Geometry: final body of the model. Coordinates: model frame, mm. Face numbers are marked on the shaded views. A direction names the side the tool comes from. Round coordinates to 2 decimals unless told otherwise and drop trailing zeros. Order: outer loops, then holes, each group sorted by start corner. A loop starts at its lowest first (then second) coordinate and runs counter-clockwise, first axis right, second up. Notation, with made-up numbers: (88, 80) -> (117, 80) arc R8 ccw to (117, 89) -> close; hole circle Ø8 at (41.25, -14.75). An arc over 180 degrees is marked (long way). Put each result on its own line as item: value.
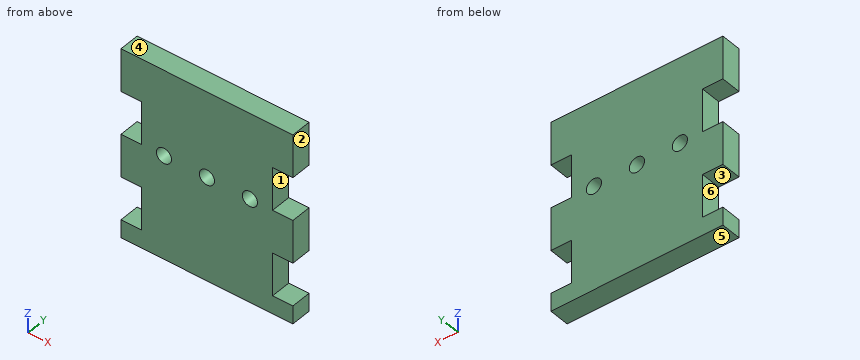
```python
from build123d import *

# Parameters (mm, degrees)
SKETCH1_W            = 50.8
SKETCH1_H            = 56.134
MAIN_DEPTH           = 6
SKETCH2_W            = 6
SKETCH2_H            = 12.7
ACRYLIC_MOUNTS_DEPTH = 39.326446339
SKETCH3_R            = 2.2479
CUT_EXTRUDE1_DEPTH   = 39.326446339


with BuildPart() as part:
    # Sketch1 → Main (new body)
    with BuildSketch(Plane(origin=(0, 0, 0), x_dir=(1, 0, 0), z_dir=(0, 1, 0))):
        Rectangle(SKETCH1_W, SKETCH1_H)
    extrude(amount=MAIN_DEPTH)

    # Sketch2 → Acrylic Mounts (cut, through all)
    with BuildSketch(Plane(origin=(0, 6, 0), x_dir=(1, 0, 0), z_dir=(0, 1, 0))):
        with Locations((-22.4, -9.017)):
            Rectangle(SKETCH2_W, SKETCH2_H)
        with Locations((-22.4, 16.383)):
            Rectangle(SKETCH2_W, SKETCH2_H)
        with Locations((22.4, 16.383)):
            Rectangle(SKETCH2_W, SKETCH2_H)
        with Locations((22.4, -9.017)):
            Rectangle(SKETCH2_W, SKETCH2_H)
    extrude(amount=-ACRYLIC_MOUNTS_DEPTH, mode=Mode.SUBTRACT)

    # Sketch3 → Cut-Extrude1 (cut, through all)
    with BuildSketch(Plane(origin=(0, 0, 0), x_dir=(-1, 0, 0), z_dir=(0, -1, 0))):
        with Locations(Location((12.7, -2.667, 0), (0, 0, 90))):
            Circle(SKETCH3_R)
        with Locations(Location((-12.7, -2.667, 0), (0, 0, 90))):
            Circle(SKETCH3_R)
        with Locations(Location((0, -2.667, 0), (0, 0, 90))):
            Circle(SKETCH3_R)
    extrude(amount=-CUT_EXTRUDE1_DEPTH, mode=Mode.SUBTRACT)


solid = part.part
```
1. Draft query along Z for the marked faces 4, 5 and 6. Return one class per face: +Z half, -Z half, draft (parallel to the pull), parting line (faces both ways), or undercut.
Ans:
face 4: +Z half
face 5: -Z half
face 6: undercut
2. Cut plane B-B on y = 1.05. Return loops of the section in (x, z), and give its area (3 significant figures).
Ans:
outline: (-25.4, -28.07) -> (25.4, -28.07) -> (25.4, -22.73) -> (19.4, -22.73) -> (19.4, -10.03) -> (25.4, -10.03) -> (25.4, 2.67) -> (19.4, 2.67) -> (19.4, 15.37) -> (25.4, 15.37) -> (25.4, 28.07) -> (-25.4, 28.07) -> (-25.4, 15.37) -> (-19.4, 15.37) -> (-19.4, 2.67) -> (-25.4, 2.67) -> (-25.4, -10.03) -> (-19.4, -10.03) -> (-19.4, -22.73) -> (-25.4, -22.73) -> close; hole circle Ø4.5 at (-12.7, 2.67); hole circle Ø4.5 at (0, 2.67); hole circle Ø4.5 at (12.7, 2.67)
area: 2,500 mm²
3. Contact query for flat-ended pins moving along their axis: P1, Ø1.8, axis at y = 4.5, z = 6.5, coming from the -X side; P2, Ø1.8, axis at y = 3.5, z = -18, coming from the +X side. Output: stop coordinate, or through.
Ans:
P1: x = -19.4
P2: x = 19.4
4. Set-up query: the marked faces 1, 2 and 3. Return all of +Z, -Z, +X, -X, +Y, -Y with unobstructed straight access to the full face (end or side cutting, diameter ignored); none if empty.
Ans:
face 1: +X, +Y, -Y
face 2: +Z, -Z, +X, +Y, -Y
face 3: -X, +Y, -Y
5. Material intervals for probe 1 along Z at (x, y) = (22, 0.4); probe 2 along X at (y, z) = (1.4, 7); probe 3 along Z at (x, y) = (-0.5, 5.65), sorted ascending.
Ans:
probe 1: -28.07 to -22.73, -10.03 to 2.67, 15.37 to 28.07
probe 2: -19.4 to 19.4
probe 3: -28.07 to 0.48, 4.86 to 28.07
6. Cut plane A-A on x = -12.7. Return loops of the section in (y, z).
Ans:
outline: (0, -28.07) -> (6, -28.07) -> (6, 0.42) -> (0, 0.42) -> close; (0, 4.91) -> (6, 4.91) -> (6, 28.07) -> (0, 28.07) -> close
7. Cut plane C-C on z = -15.5. Return loops of the section in (x, y).
Ans:
outline: (-19.4, 0) -> (19.4, 0) -> (19.4, 6) -> (-19.4, 6) -> close
